from build123d import *

# Parameters (mm, degrees)
SKETCH_1_W          = 32.5
SKETCH_1_H          = 109
EXTRUDE_1_DEPTH     = 3
FILLET_2_R          = 3
SKETCH_2_W          = 26
SKETCH_2_H          = 103
EXTRUDE_2_DEPTH     = 15
SKETCH_4_R          = 10
EXTRUDE_3_DEPTH     = 8.5
CUT_EXTRUDE_1_DEPTH = 10
SKETCH_6_W          = 20
SKETCH_6_H          = 12
CUT_EXTRUDE_2_DEPTH = 5
CUT_EXTRUDE_2_DRAFT = -15
SKETCH_7_W          = 20
SKETCH_7_H          = 10
REVOLVE_1_ANGLE     = 15
FILLET_START        = -47
FILLET_3_DEPTH      = 12
FILLET_START_2      = -11
FILLET_3_2_DEPTH    = 22
SKETCH_8_R          = 6
CUT_EXTRUDE_3_DEPTH = 64.76973092


with BuildPart() as part:
    # 草圖1 → 伸長1 (new body)
    with BuildSketch(Plane.XY):
        Rectangle(SKETCH_1_W, SKETCH_1_H)
    extrude(amount=EXTRUDE_1_DEPTH)

    # 圓角2
    fillet_2_edges = [part.edges().sort_by_distance(p)[0] for p in [
        (-16.25, 0, 3),
        (16.25, 0, 3),
        (0, -54.5, 3),
        (0, 54.5, 3),
    ]]
    fillet(fillet_2_edges, radius=FILLET_2_R - 0.0001)  # a hair under: the kernel refuses the full size

    # 草圖2 → 伸長2 (add)
    with BuildSketch(Plane(origin=(0, 0, 0), x_dir=(-1, 0, 0), z_dir=(0, 0, -1))):
        Rectangle(SKETCH_2_W, SKETCH_2_H)
    extrude(amount=EXTRUDE_2_DEPTH)

    # 草圖4 → 伸長3 (add)
    with BuildSketch(Plane(origin=(0, 0, -15), x_dir=(-1, 0, 0), z_dir=(0, 0, -1))):
        with Locations((0, 38.5)):
            Circle(SKETCH_4_R)
    extrude(amount=EXTRUDE_3_DEPTH)

    # 草圖5 → 除料-伸長1 (cut)
    with BuildSketch(Plane.XY.offset(3)):
        with BuildLine():
            Line((-10, 38.5), (-10, -36.5))
            Line((-10, -36.5), (10, -36.5))
            Line((10, -36.5), (10, 38.5))
            ThreePointArc((10, 38.5), (0, 48.5), (-10, 38.5))
        make_face()
    extrude(amount=-CUT_EXTRUDE_1_DEPTH, mode=Mode.SUBTRACT)


with BuildPart() as cut_extrude_2_tool:
    # 草圖6 → 除料-伸長2 (with draft: the straight prism first)
    with BuildSketch(Plane.XY.offset(-7)):
        with Locations((0, -30.5)):
            Rectangle(SKETCH_6_W, SKETCH_6_H)
    extrude(amount=-CUT_EXTRUDE_2_DEPTH)
    # 除料-伸長2: the draft: its side faces are tilted about the plane it starts from
    cut_extrude_2_sides = [cut_extrude_2_tool.faces().sort_by_distance(p)[0] for p in [
        (0, -36.5, -9.5),
        (10, -30.5, -9.5),
        (0, -24.5, -9.5),
        (-10, -30.5, -9.5),
    ]]
    draft(cut_extrude_2_sides, Plane.XY.offset(-7), CUT_EXTRUDE_2_DRAFT)


with BuildPart() as part_1:
    add(part.part)

    # 除料-伸長2: cut by cut_extrude_2_tool
    add(cut_extrude_2_tool.part, mode=Mode.SUBTRACT)

    # 草圖7 → 旋轉1 (revolve)
    with BuildSketch(Plane.XY.offset(3)):
        with Locations((0, -41.5)):
            Rectangle(SKETCH_7_W, SKETCH_7_H)
    revolve(axis=Axis((-10, -36.5, 3), (-1, 0, 0)), revolution_arc=REVOLVE_1_ANGLE)

    # 圓角3: read off the stored shape, not the designer's step
    # 圓角3 outline → 圓角3 (cut)
    with BuildSketch(Plane(origin=(0, 0, 0), x_dir=(1, 0, 0), z_dir=(0, 0.9659258262890682, -0.2588190451025211)).offset(FILLET_START)):
        with BuildLine():
            ThreePointArc((10, 7.049117667), (9.853553391, 6.695564276), (9.5, 6.549117667))
            Line((9.5, 6.549117667), (10, 6.549117667))
            Line((10, 6.549117667), (10, 7.049117667))
        make_face()
        with BuildLine():
            ThreePointArc((-9.5, 6.549117667), (-9.853553391, 6.695564276), (-10, 7.049117667))
            Line((-10, 7.049117667), (-10, 6.549117667))
            Line((-10, 6.549117667), (-9.5, 6.549117667))
        make_face()
    extrude(amount=FILLET_3_DEPTH, mode=Mode.SUBTRACT)

    # Fillet 3 2 outline → Fillet 3 2 (cut)
    with BuildSketch(Plane.YZ.offset(FILLET_START_2)):
        with BuildLine():
            ThreePointArc((-46.387024756, 4.498913432), (-45.945734853, 5.185884966), (-45.139503235, 5.314947915))
            Line((-45.139503235, 5.314947915), (-46.159258263, 5.588190451))
            ThreePointArc((-46.159258263, 5.588190451), (-46.288305577, 5.04672273), (-46.387024756, 4.498913432))
        make_face()
    extrude(amount=FILLET_3_2_DEPTH, mode=Mode.SUBTRACT)

    # 草圖8 → 除料-伸長3 (cut, through all)
    with BuildSketch(Plane(origin=(0, 0, -23.5), x_dir=(-1, 0, 0), z_dir=(0, 0, -1))):
        with Locations((0, 38.5)):
            Circle(SKETCH_8_R)
    extrude(amount=-CUT_EXTRUDE_3_DEPTH, mode=Mode.SUBTRACT)


solid = part_1.part
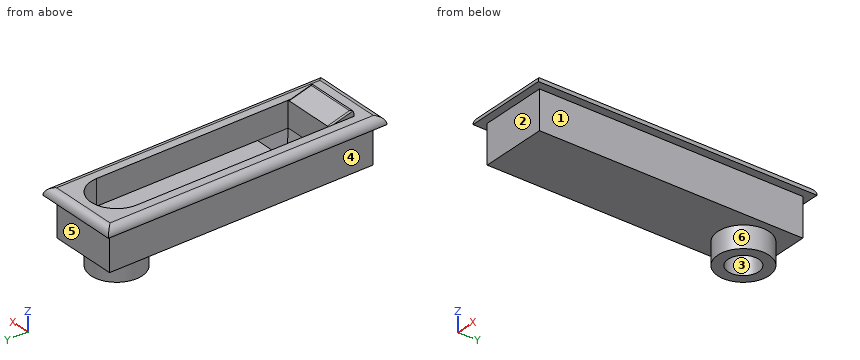
The model under review builds one solid part; all positions refer to its coordinate system, in mm. Face numbers are marked on the shaded views. A direction names the side the tool comes from. Coordinates: 2 decimals unless noted, no trailing zeros. Loops run counter-clockwise (first coordinate to the right, second up) from the corner with the lowest first, then second, coordinate; pieces in that order, holes last. Notation, with made-up numbers: (87.25, 15.25) -> (113.25, 15.25) arc R21 cw to (113.25, 36.25) -> close; hole circle Ø6 at (71.25, 21). An arc over 180 degrees is marked (long way). Use a Markdown table: item, result. Add a question column.
1. To check wall thickness, follow line 1 (Y direction, x = 0, z = -15.75); line 2 (Y direction, x = 0, z = -14); line 3 (X direction, y = -24.5, z = -5.5). State the ranges of each line that lie inside material, in increasing order.
2. Draft analysis for pull direction X (two halves, no side actions). For the marked faces 1, 2 and 3, state which applies: pulls with the +X half, pulls with the -X half, needs draft (parallel to the pull), parting line crosses it, or undercut.
3. Clearance check with flat-ended pins moving along their axes: pin 1 Ø11 at (y, z) = (10, -1.5) entering from -X; pin 2 Ø3 at (y, z) = (15, -14) entering from +X; pin 3 Ø3 at (x, y) = (3.5, -31) entering from +Z; pin 4 Ø2 at (y, z) = (40, -4.5) entering from -X. State where each tip first meets the part, or that it passes through.
4. Machinability: for the marked faces 4, 5 and 6, which of the approach directions +Z, -Z, +X, -X, +Y, -Y give a long, thin tool a straight path to every point of the face, cutting with its end or side? Answer none if there is none.
5. Add section C-C on z = -9.5. Write out the cut boundary in (x, y), plus the area to 3 significant figures.
Returned:
| question | item | result |
|---|---|---|
| 1 | line 1 | y = 28.5 to 32.5, 44.5 to 48.5 |
| 1 | line 2 | y = -51.5 to 32.5, 44.5 to 51.5 |
| 1 | line 3 | x = -13 to -10, 10 to 13 |
| 2 | face 1 | pulls with the +X half |
| 2 | face 2 | needs draft |
| 2 | face 3 | undercut |
| 3 | pin 1 | stops at x = -16.25 |
| 3 | pin 2 | stops at x = 13 |
| 3 | pin 3 | stops at z = -12 |
| 3 | pin 4 | stops at x = -13 |
| 4 | face 4 | -Z, -X, +Y, -Y |
| 4 | face 5 | -Z, +X, -X, +Y |
| 4 | face 6 | -Z |
| 5 | outline | (-13, -51.5) -> (13, -51.5) -> (13, 51.5) -> (-13, 51.5) -> close; hole (-9.33, -35.83) -> (9.33, -35.83) -> (9.33, -25.17) -> (-9.33, -25.17) -> close; hole circle Ø12 at (0, 38.5) |
| 5 | area | 2,370 mm² |
